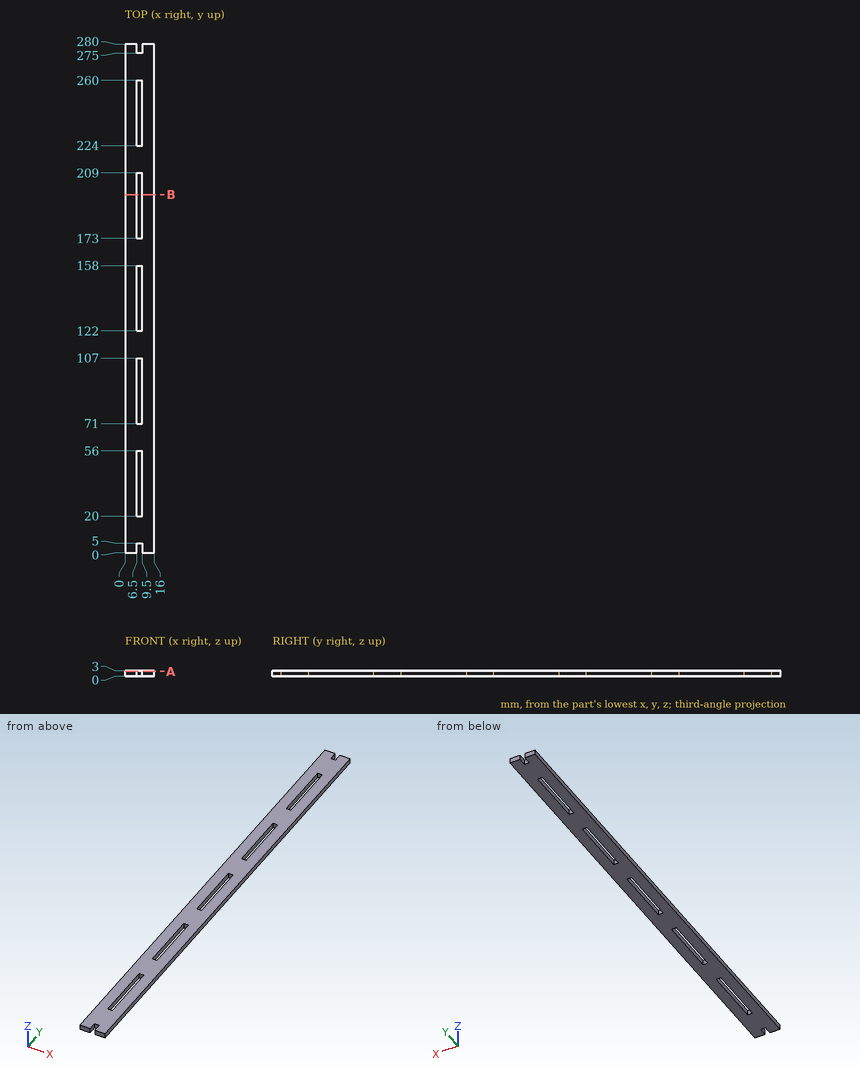
Job drawing, mm, ordinate dimensions from the low corner. One solid piece. Give positions to 0.01 mm unless a question says otherwise; leave off trailing zeros. Loops run counter-clockwise (first coordinate to the right, second up) from the corner with the lowest first, then second, coordinate; pieces in that order, holes last. Notation, with made-up numbers: M 86,38 L 111,38 A19 cw 111,56 Z; hole C 53,14.25 d7. An arc over 180 degrees is marked long. Put each result on its own line as item: value. Start each with the question number.
1) Probe probe 1 along Y at (x, z) = (7.25, 0.3); probe 2 along X at (y, z) = (148.5, 2.25). List the from-to ranges inside material, lowest first.
2) Saw through at A-A (z = 2.5). State how many separate pieces and enclosed holes the cut face has, then the cut area to 3 significant figures.
3) Saw through at B-B (y = 197). List the corners of the cut face in (x, z), then the cut area to 3 significant figures.
4) Flat gauge pin, fed straight in: pin 1 (1.5 mm diameter, centred on x = 8, z = 1, fed in from +Y). Where does the tip first touch, or does it go through?
Numbers:
1. probe 1: 5 to 20, 56 to 71, 107 to 122, 158 to 173, 209 to 224, 260 to 275
1. probe 2: 0 to 6.5, 9.5 to 16
2. separate pieces: 1
2. enclosed holes: 5
2. area: 3,910 mm^2
3. outline: M 0,0 L 6.5,0 L 6.5,3 L 0,3 Z; M 9.5,0 L 16,0 L 16,3 L 9.5,3 Z
3. area: 39.0 mm^2
4. pin 1: y = 275
